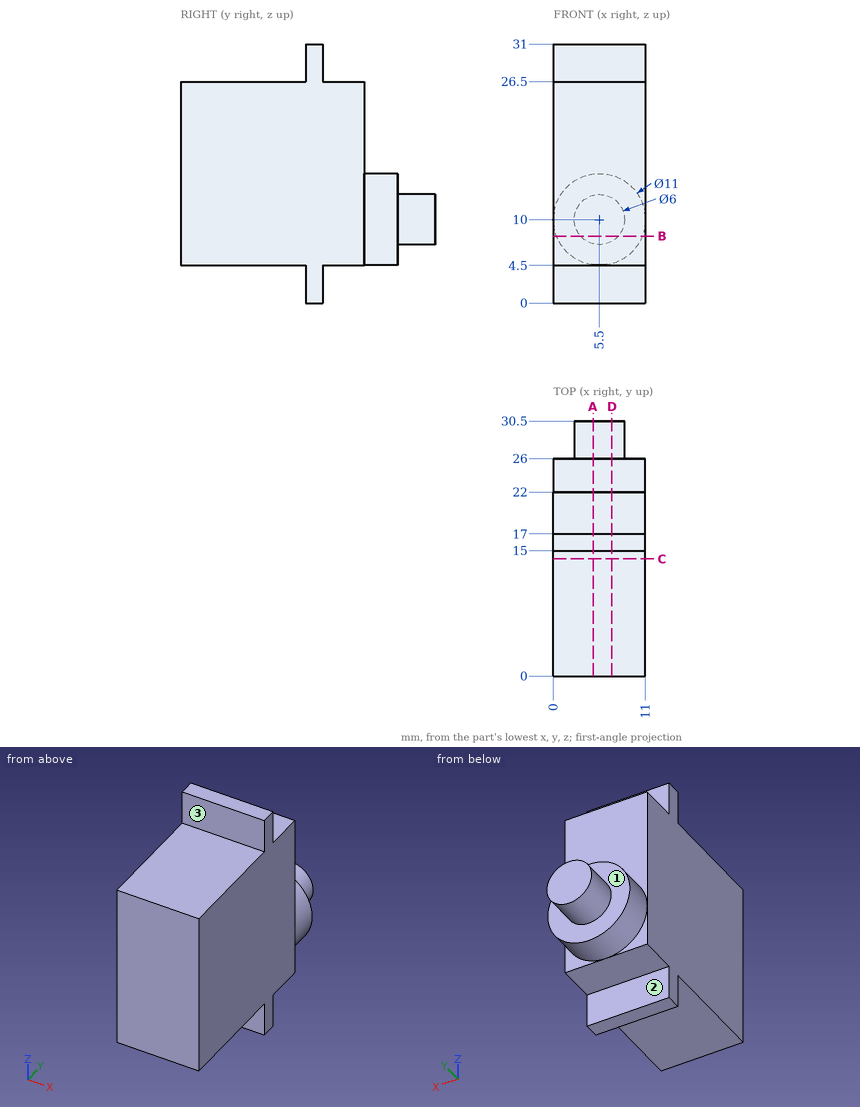
Answer from the drawing. Dimensions are ordinates in mm from the lowest x, y and z of the part. A direction names the side the tool comes from. Give positions to 0.01 mm unless a question says otherwise; leave off trailing zeros. Order: outer loops, then holes, each group sorted by start corner. A loop starts at its lowest first (then second) coordinate and runs counter-clockwise, first axis right, second up.
Item 1: The part is cut by section C-C, the plane y = 14. Give the vertices of the cut face in (x, z), and give its area (3 significant figures).
From the geometry:
outline: (0, 4.5) - (11, 4.5) - (11, 26.5) - (0, 26.5) - close
area: 242 mm2
Item 2: Given pin 1 Ø2 at (x, z) = (7.5, 2.5) entering from +Y; pin 2 Ø1 at (x, y) = (1.5, 9.5) entering from -Z; pin 3 Ø5.5 at (x, y) = (4, 19.5) entering from -Z; pin 4 Ø3.5 at (x, z) = (8, 2) entering from -Y, each flat-ended and moving along its own axis, determine where each tip first touches the part or whether it passes through.
From the geometry:
pin 1: stops at y = 17
pin 2: stops at z = 4.5
pin 3: stops at z = 0
pin 4: stops at y = 15
Item 3: The part is cut by section A-A, the plane x = 4.75. Give the vertices of the cut face in (y, z).
From the geometry:
outline: (0, 4.5) - (15, 4.5) - (15, 0) - (17, 0) - (17, 4.5) - (22, 4.5) - (22, 4.55) - (26, 4.55) - (26, 7.1) - (30.5, 7.1) - (30.5, 12.9) - (26, 12.9) - (26, 15.45) - (22, 15.45) - (22, 26.5) - (17, 26.5) - (17, 31) - (15, 31) - (15, 26.5) - (0, 26.5) - close
Item 4: The part is cut by section B-B, the plane z = 8. Give the vertices of the cut face in (x, y).
From the geometry:
outline: (0, 0) - (11, 0) - (11, 22) - (10.62, 22) - (10.62, 26) - (7.74, 26) - (7.74, 30.5) - (3.26, 30.5) - (3.26, 26) - (0.38, 26) - (0.38, 22) - (0, 22) - close
Item 5: Find the intervals of material crossed by probe 1 along Y at (x, z) = (8.5, 20); probe 2 along Z at (x, y) = (9.5, 6); probe 3 along Y at (x, z) = (4.5, 14), in increasing order.
From the geometry:
probe 1: y = 0 to 22
probe 2: z = 4.5 to 26.5
probe 3: y = 0 to 26
Item 6: The part is cut by section D-D, the plane x = 7. Give the vertices of the cut face in (y, z), and give its area (3 significant figures).
From the geometry:
outline: (0, 4.5) - (15, 4.5) - (15, 0) - (17, 0) - (17, 4.5) - (22, 4.5) - (22, 4.71) - (26, 4.71) - (26, 7.4) - (30.5, 7.4) - (30.5, 12.6) - (26, 12.6) - (26, 15.29) - (22, 15.29) - (22, 26.5) - (17, 26.5) - (17, 31) - (15, 31) - (15, 26.5) - (0, 26.5) - close
area: 568 mm2
Item 7: Which of the six approach directions +Z, -Z, +X, -X, +Y, -Y give full straight-line access (tool end or side, diameter ignored) to the marked faces 1, 2 and 3?
From the geometry:
face 1: +Y
face 2: -Z, +X, -X, +Y
face 3: +Z, +X, -X, -Y
